Design review of the part built by this model. Coordinates are the model's own, in mm. Face numbers are marked on the shaded views. A direction names the side the tool comes from. Coordinates: 2 decimals unless noted, no trailing zeros. Loops run counter-clockwise (first coordinate to the right, second up) from the corner with the lowest first, then second, coordinate; pieces in that order, holes last. Notation, with made-up numbers: (75.5, -39) -> (98.5, -39) arc R16 ccw to (98.5, -34) -> close; hole circle Ø6 at (63.25, 5). An arc over 180 degrees is marked (long way). Answer in a Markdown table with one row per item.
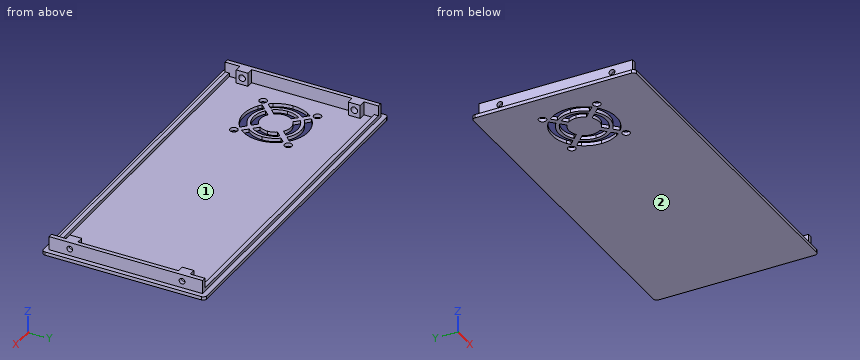
```python
from build123d import *

# Parameters (mm, degrees)
P_DORYS_W                                         = 201
P_DORYS_H                                         = 96
P_IDAT_VYSUNUT_M1_DEPTH                           = 2
ZAOBLIT1_R                                        = 2
SKICA2_W                                          = 195.2
SKICA2_H                                          = 90.2
SKICA2_W_2                                        = 190.2
SKICA2_H_2                                        = 85.2
SKICA2_W_3                                        = 4
SKICA2_H_3                                        = 7
P_IDAT_VYSUNUT_M2_DEPTH                           = 2
P_IDAT_VYSUNUT_M3_DEPTH                           = 6
V_LCOV_ZAHLOUBEN_PRO_M6_ROUBY_S_V_LCO_D           = 3.4
V_LCOV_ZAHLOUBEN_PRO_M6_ROUBY_S_V_LCO_DEPTH       = 9.4
V_LCOV_ZAHLOUBEN_PRO_M6_ROUBY_S_V_LCO_CBORE_D     = 3.9
V_LCOV_ZAHLOUBEN_PRO_M6_ROUBY_S_V_LCO_CBORE_DEPTH = 4
SKICA7_R                                          = 2.25
ODEBRAT_VYSUNUT_M1_DEPTH                          = 6


with BuildPart() as part:
    # půdorys → Přidat vysunutím1 (new body)
    with BuildSketch(Plane.XY):
        Rectangle(P_DORYS_W, P_DORYS_H)
    extrude(amount=P_IDAT_VYSUNUT_M1_DEPTH)

    # Zaoblit1
    zaoblit1_edges = [part.edges().sort_by_distance(p)[0] for p in [
        (100.5, -48, 1),
        (-100.5, -48, 1),
        (-100.5, 48, 1),
        (100.5, 48, 1),
    ]]
    fillet(zaoblit1_edges, radius=ZAOBLIT1_R)

    # Skica2 → Přidat vysunutím2 (add)
    # profile 1 of 5: a face of its own
    with BuildSketch(Plane.XY.offset(2)):
        Rectangle(SKICA2_W, SKICA2_H)
        Rectangle(SKICA2_W_2, SKICA2_H_2, mode=Mode.SUBTRACT)
    # profile 2 of 5: a face of its own
    with BuildSketch(Plane.XY.offset(2)):
        with Locations((93.1, -33)):
            Rectangle(SKICA2_W_3, SKICA2_H_3)
    # profile 3 of 5: a face of its own
    with BuildSketch(Plane.XY.offset(2)):
        with Locations((93.1, 33)):
            Rectangle(SKICA2_W_3, SKICA2_H_3)
    # profile 4 of 5: a face of its own
    with BuildSketch(Plane.XY.offset(2)):
        with Locations((-93.1, 33)):
            Rectangle(SKICA2_W_3, SKICA2_H_3)
    # profile 5 of 5: a face of its own
    with BuildSketch(Plane.XY.offset(2)):
        with Locations((-93.1, -33)):
            Rectangle(SKICA2_W_3, SKICA2_H_3)
    extrude(amount=P_IDAT_VYSUNUT_M2_DEPTH)

    # Skica3 → Přidat vysunutím3 (add)
    with BuildSketch(Plane.XY.offset(4)):
        Polygon((95.1, 45.1), (95.1, 36.5), (91.1, 36.5), (91.1, 29.5), (95.1, 29.5), (95.1, -29.5), (91.1, -29.5), (91.1, -36.5), (95.1, -36.5), (95.1, -45.1), (97.6, -45.1), (97.6, 45.1), align=None)
        Polygon((-95.1, -45.1), (-95.1, -36.5), (-91.1, -36.5), (-91.1, -29.5), (-95.1, -29.5), (-95.1, 29.5), (-91.1, 29.5), (-91.1, 36.5), (-95.1, 36.5), (-95.1, 45.1), (-97.6, 45.1), (-97.6, -45.1), align=None)
    extrude(amount=P_IDAT_VYSUNUT_M3_DEPTH)

    # Válcové zahloubení pro M6 šrouby s válcovou hlavou zaoblenou1
    with Locations(Plane(origin=(-91.1, 33, 6), x_dir=(0, 0, 1), z_dir=(1, 0, 0))):
        with Locations((0, 0), (0, 66)):
            v_lcov_zahlouben_pro_m6_rouby_s_v_lco = CounterBoreHole(V_LCOV_ZAHLOUBEN_PRO_M6_ROUBY_S_V_LCO_D / 2, V_LCOV_ZAHLOUBEN_PRO_M6_ROUBY_S_V_LCO_CBORE_D / 2, V_LCOV_ZAHLOUBEN_PRO_M6_ROUBY_S_V_LCO_CBORE_DEPTH, depth=V_LCOV_ZAHLOUBEN_PRO_M6_ROUBY_S_V_LCO_DEPTH)

    # Zrcadlit1: Válcové zahloubení pro M6 šrouby s válcovou hlavou zaoblenou1 across plane
    add(v_lcov_zahlouben_pro_m6_rouby_s_v_lco.mirror(Plane(origin=(0, 0, 0), x_dir=(0, 0, 1), z_dir=(1, 0, 0))), mode=Mode.SUBTRACT)

    # Skica7 → Odebrat vysunutím1 (cut)
    with BuildSketch(Plane(origin=(0, 0, 0), x_dir=(-1, 0, 0), z_dir=(0, 0, -1))):
        with BuildLine():
            Line((82.5, 10.246950766), (82.5, 0))
            Line((82.5, 0), (85.5, 0))
            ThreePointArc((85.5, 0), (84.734582529, 5.338539126), (82.5, 10.246950766))
        make_face()
        with BuildLine():
            Line((85.5, 0), (82.5, 0))
            Line((82.5, 0), (82.5, -10.246950766))
            ThreePointArc((82.5, -10.246950766), (84.734582529, -5.338539126), (85.5, 0))
        make_face()
        with BuildLine():
            ThreePointArc((78.171770833, 9.421770833), (80.643489005, 4.996170409), (81.5, 0))
            Line((81.5, 0), (82.5, 0))
            Line((82.5, 0), (82.5, 10.246950766))
            ThreePointArc((82.5, 10.246950766), (81.789681929, 11.279433784), (81.0128443, 12.2628443))
            Line((81.0128443, 12.2628443), (78.171770833, 9.421770833))
        make_face()
        with BuildLine():
            ThreePointArc((57.078229167, 11.671770833), (66.586420622, 14.999751047), (76.055634012, 11.562433076))
            Line((76.055634012, 11.562433076), (78.908692733, 14.38834058))
            ThreePointArc((78.908692733, 14.38834058), (77.856447821, 15.232566852), (76.746950766, 16))
            Line((76.746950766, 16), (56.253049234, 16))
            ThreePointArc((56.253049234, 16), (55.220566216, 15.289681929), (54.2371557, 14.5128443))
            Line((54.2371557, 14.5128443), (57.078229167, 11.671770833))
        make_face()
        with BuildLine():
            Line((56.253049234, 16), (76.746950766, 16))
            ThreePointArc((76.746950766, 16), (66.5, 19), (56.253049234, 16))
        make_face()
        with BuildLine():
            ThreePointArc((51.5, 0), (52.356510995, 4.996170409), (54.828229167, 9.421770833))
            Line((54.828229167, 9.421770833), (51.9871557, 12.2628443))
            ThreePointArc((51.9871557, 12.2628443), (51.210318071, 11.279433784), (50.5, 10.246950766))
            Line((50.5, 10.246950766), (50.5, 0))
            Line((50.5, 0), (51.5, 0))
        make_face()
        with BuildLine():
            Line((50.5, 0), (50.5, 10.246950766))
            ThreePointArc((50.5, 10.246950766), (48.265417471, 5.338539126), (47.5, 0))
            Line((47.5, 0), (50.5, 0))
        make_face()
        with BuildLine():
            Line((50.5, -10.246950766), (50.5, 0))
            Line((50.5, 0), (47.5, 0))
            ThreePointArc((47.5, 0), (48.265417471, -5.338539126), (50.5, -10.246950766))
        make_face()
        with BuildLine():
            Line((51.993667632, -12.2705469), (54.846726353, -9.444639395))
            ThreePointArc((54.846726353, -9.444639395), (52.361416183, -5.010034695), (51.5, 0))
            Line((51.5, 0), (50.5, 0))
            Line((50.5, 0), (50.5, -10.246950766))
            ThreePointArc((50.5, -10.246950766), (51.213312525, -11.283491748), (51.993667632, -12.2705469))
        make_face()
        with BuildLine():
            Line((78.7628443, -14.5128443), (75.921770833, -11.671770833))
            ThreePointArc((75.921770833, -11.671770833), (66.5, -15), (57.078229167, -11.671770833))
            Line((57.078229167, -11.671770833), (54.2371557, -14.5128443))
            ThreePointArc((54.2371557, -14.5128443), (55.220566216, -15.289681929), (56.253049234, -16))
            Line((56.253049234, -16), (76.746950766, -16))
            ThreePointArc((76.746950766, -16), (77.779433784, -15.289681929), (78.7628443, -14.5128443))
        make_face()
        with BuildLine():
            ThreePointArc((56.253049234, -16), (66.5, -19), (76.746950766, -16))
            Line((76.746950766, -16), (56.253049234, -16))
        make_face()
        with BuildLine():
            Line((82.5, 0), (81.5, 0))
            ThreePointArc((81.5, 0), (80.643489005, -4.996170409), (78.171770833, -9.421770833))
            Line((78.171770833, -9.421770833), (81.0128443, -12.2628443))
            ThreePointArc((81.0128443, -12.2628443), (81.789681929, -11.279433784), (82.5, -10.246950766))
            Line((82.5, -10.246950766), (82.5, 0))
        make_face()
        with BuildLine():
            ThreePointArc((76.748287511, -7.998287511), (78.792838111, -4.229199828), (79.5, 0))
            Line((79.5, 0), (75.5, 0))
            ThreePointArc((75.5, 0), (75.087741676, -2.692711071), (73.888734908, -5.138734908))
            Line((73.888734908, -5.138734908), (76.748287511, -7.998287511))
        make_face()
        with BuildLine():
            ThreePointArc((58.501712489, -10.248287511), (66.5, -13), (74.498287511, -10.248287511))
            Line((74.498287511, -10.248287511), (71.638734908, -7.388734908))
            ThreePointArc((71.638734908, -7.388734908), (66.5, -9), (61.361265092, -7.388734908))
            Line((61.361265092, -7.388734908), (58.501712489, -10.248287511))
        make_face()
        with BuildLine():
            ThreePointArc((53.5, 0), (54.213544679, -4.247707105), (56.275848561, -8.02911747))
            Line((56.275848561, -8.02911747), (59.145152054, -5.187119788))
            ThreePointArc((59.145152054, -5.187119788), (57.921141349, -2.720879314), (57.5, 0))
            Line((57.5, 0), (53.5, 0))
        make_face()
        with BuildLine():
            Line((59.111265092, 5.138734908), (56.251712489, 7.998287511))
            ThreePointArc((56.251712489, 7.998287511), (54.207161889, 4.229199828), (53.5, 0))
            Line((53.5, 0), (57.5, 0))
            ThreePointArc((57.5, 0), (57.912258324, 2.692711071), (59.111265092, 5.138734908))
        make_face()
        with BuildLine():
            Line((71.757208311, 7.304913468), (74.626511804, 10.146911151))
            ThreePointArc((74.626511804, 10.146911151), (66.581729181, 12.999743088), (58.501712489, 10.248287511))
            Line((58.501712489, 10.248287511), (61.361265092, 7.388734908))
            ThreePointArc((61.361265092, 7.388734908), (66.572563732, 8.999707468), (71.757208311, 7.304913468))
        make_face()
        with BuildLine():
            Line((75.5, 0), (79.5, 0))
            ThreePointArc((79.5, 0), (78.792838111, 4.229199828), (76.748287511, 7.998287511))
            Line((76.748287511, 7.998287511), (73.888734908, 5.138734908))
            ThreePointArc((73.888734908, 5.138734908), (75.087741676, 2.692711071), (75.5, 0))
        make_face()
        with Locations((50.5, -16)):
            Circle(SKICA7_R)
        with Locations((82.5, -16)):
            Circle(SKICA7_R)
        with Locations((82.5, 16)):
            Circle(SKICA7_R)
        with Locations((50.5, 16)):
            Circle(SKICA7_R)
    extrude(amount=-ODEBRAT_VYSUNUT_M1_DEPTH, mode=Mode.SUBTRACT)


solid = part.part
```
(1) Take a section at C-C on z = 6. Count the separate pieces of the cut face and the enclosed holes in it, and give its area (3 significant figures).
Evaluation:
| item | result |
|---|---|
| separate pieces | 6 |
| enclosed holes | 0 |
| area | 467 mm² |
(2) For pin 1 (1 mm diameter, centred on x = 6.5, y = -30.5, fed in from -Z); pin 2 (4 mm diameter, centred on y = 14.5, z = 6.5, fed in from -X); pin 3 (3 mm diameter, centred on x = -92.5, z = 7, fed in from +Y); pin 4 (1.2 mm diameter, centred on x = -94, z = 6, fed in from -Y), all flat-tipped, find the tip position at first contact; note any pin that passes through.
Evaluation:
| item | result |
|---|---|
| pin 1 | stops at z = 0 |
| pin 2 | stops at x = -97.6 |
| pin 3 | stops at y = 36.5 |
| pin 4 | stops at y = -36.5 |
(3) Take a section at A-A on y = 38.5. Give the boundary of the cut face in (x, z), and give its area (3 significant figures).
Evaluation:
| item | result |
|---|---|
| outline | (-100.5, 0) -> (100.5, 0) -> (100.5, 2) -> (97.6, 2) -> (97.6, 10) -> (95.1, 10) -> (95.1, 2) -> (-95.1, 2) -> (-95.1, 10) -> (-97.6, 10) -> (-97.6, 2) -> (-100.5, 2) -> close |
| area | 442 mm² |
(4) Tool access review of the marked faces 1 and 2: name each direction out of +Z, -Z, +X, -X, +Y, -Y from which nothing blocks a thin tool from reaching the whole face with its end or side.
Evaluation:
| item | result |
|---|---|
| face 1 | +Z |
| face 2 | -Z, +X, -X, +Y, -Y |
(5) To check wall thickness, follow probe 1 along Y at (x, z) = (-94.1, 6); probe 2 along Y at (x, z) = (-82.5, 0.9); probe 3 along Y at (x, z) = (-96.6, 6). State the ranges of each line that lie inside material, in increasing order.
Evaluation:
| item | result |
|---|---|
| probe 1 | y = -36.5 to -34.95, -31.05 to -29.5, 29.5 to 31.05, 34.95 to 36.5 |
| probe 2 | y = -48 to -18.25, -13.75 to -10.25, 10.25 to 13.75, 18.25 to 48 |
| probe 3 | y = -45.1 to -34.7, -31.3 to 31.3, 34.7 to 45.1 |
(6) Take a section at B-B on x = 12.5. Give the boundary of the cut face in (y, z).
Evaluation:
| item | result |
|---|---|
| outline | (-48, 0) -> (48, 0) -> (48, 2) -> (45.1, 2) -> (45.1, 4) -> (42.6, 4) -> (42.6, 2) -> (-42.6, 2) -> (-42.6, 4) -> (-45.1, 4) -> (-45.1, 2) -> (-48, 2) -> close |
